Could you check a few things on this model? Use its own coordinates, in mm. Coordinates: 2 decimals unless noted, no trailing zeros. Order: outer loops, then holes, each group sorted by start corner. A loop starts at its lowest first (then second) coordinate and runs counter-clockwise, first axis right, second up. Notation, with made-up numbers: (56, 28.5) -> (80, 28.5) arc R24 ccw to (80, 53.5) -> close; hole circle Ø5 at (-35, -18.5). An arc over 180 degrees is marked (long way). Use a Markdown table: item, result. Add a question column.
1) If we section it at D-D (z = 14): Write out the boundary of the cut face in (x, y), plus the area to 3 significant figures.
2) If I drill on L1, parallel to Z at x = 2.6, y = 53; L2, parallel to Y at x = 2.7, z = 42; L3, parallel to Y at x = 2.4, z = 8.5, over which ranges is the centre line in solid material (lowest first)? Write a range as [from, to].
3) If we section it at B-B (x = 1.3): Write out the boundary of the cut face in (y, z), plus the area to 3 significant figures.
4) If we section it at C-C (y = 35.5): Write out the boundary of the cut face in (x, z).
5) If we section it at A-A (y = 53): Write out the boundary of the cut face in (x, z).
6) Will these pins go through, and if not, where does the flat tip stop? pin 1 Ø1 at (x, y) = (3, 32) entering from +Z; pin 2 Ø2 at (x, z) = (1.5, 44) entering from +Y.
```python
from build123d import *

# Parameters (mm, degrees)
F0_R     = 3
F1_DEPTH = 4


with BuildPart() as f1:
    # F0 (on Right) → F1 (new body)
    with BuildSketch(Plane.YZ):
        with BuildLine():
            Line((20, 4), (20, 0))
            Line((20, 0), (40, 0))
            Line((40, 0), (40, 4))
            Line((40, 4), (56, 4))
            Line((56, 4), (56, 19))
            Line((56, 19), (60, 19))
            Line((60, 19), (60, 35))
            Line((60, 35), (56, 35))
            Line((56, 35), (56, 50))
            Line((56, 50), (60, 50))
            Line((60, 50), (60, 54))
            ThreePointArc((60, 54), (53, 61), (46, 54))
            Line((46, 54), (46, 50))
            Line((46, 50), (4, 50))
            Line((4, 50), (4, 35))
            Line((4, 35), (0, 35))
            Line((0, 35), (0, 19))
            Line((0, 19), (4.510439, 19))
            Line((4.510439, 19), (4.510439, 4))
            Line((4.510439, 4), (20, 4))
        make_face()
        with Locations((53, 54)):
            Circle(F0_R, mode=Mode.SUBTRACT)
    extrude(amount=F1_DEPTH)


solid = f1.part
```
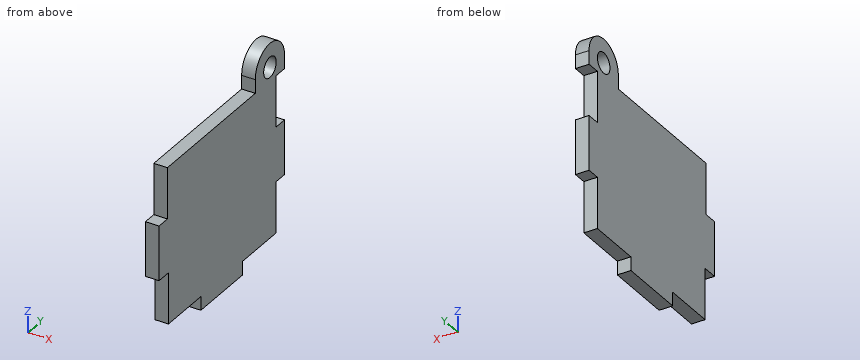
Answer sheet:
| question | item | result |
|---|---|---|
| 1 | outline | (0, 4.51) -> (4, 4.51) -> (4, 56) -> (0, 56) -> close |
| 1 | area | 206 mm2 |
| 2 | L1 | [4, 51], [57, 61] |
| 2 | L2 | [4, 56] |
| 2 | L3 | [4.51, 56] |
| 3 | outline | (0, 19) -> (4.51, 19) -> (4.51, 4) -> (20, 4) -> (20, 0) -> (40, 0) -> (40, 4) -> (56, 4) -> (56, 19) -> (60, 19) -> (60, 35) -> (56, 35) -> (56, 50) -> (60, 50) -> (60, 54) arc R7 ccw to (46, 54) -> (46, 50) -> (4, 50) -> (4, 35) -> (0, 35) -> close; hole circle Ø6 at (53, 54) |
| 3 | area | 2,700 mm2 |
| 4 | outline | (0, 0) -> (4, 0) -> (4, 50) -> (0, 50) -> close |
| 5 | outline | (0, 4) -> (4, 4) -> (4, 51) -> (0, 51) -> close; (0, 57) -> (4, 57) -> (4, 61) -> (0, 61) -> close |
| 6 | pin 1 | z = 50 |
| 6 | pin 2 | y = 56 |
